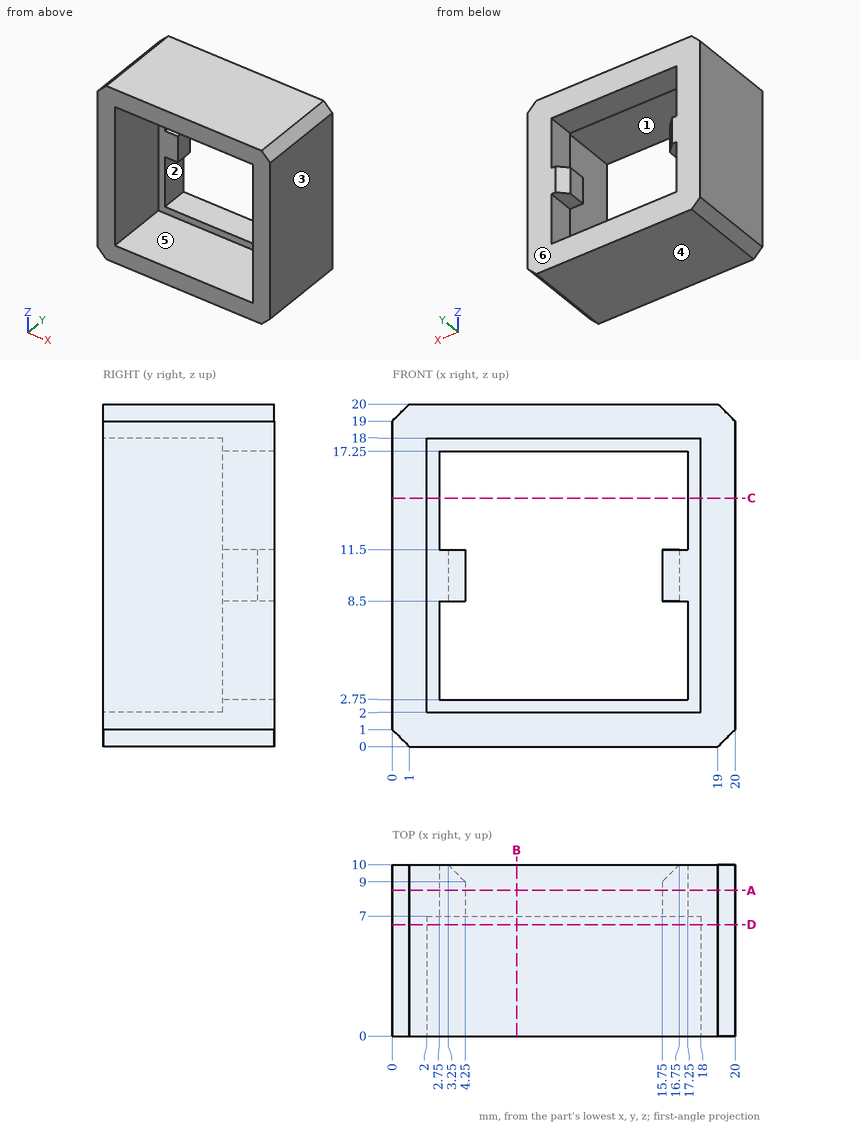
Part print with two shaded views. Sizes in mm from the minimum x, y, z corner. A direction names the side the tool comes from. Round coordinates to 2 decimals unless told otherwise and drop trailing zeros. Write each loop counter-clockwise with the first axis right and the second up, starting at its lowest first coordinate (ties: lowest second). Pieces come first, ordered by that corner, then holes. Notation, with made-up numbers: M 45,-9 L 52,-9 A18 cw 52,26 Z; hole C 66.25,77.5 d9. An arc over 180 degrees is marked long. Answer as CSV lines item,"result". Start each with the question number.
1) Mould opens along Z. For the marked faces 4, 5 and 6 say: +Z half, -Z half, draft (parallel to the pull), parting line (faces both ways), or undercut.
2) Drop a flat-ended pin along its axis: pin 1 (5 mm diameter, centred on x = 11.5, z = 12, fed in from -Y). Give the stop position or say it passes through.
3) Band-saw the part on C-C (z = 14.5). List the corners of the cut face in (x, y).
4) Band-saw the part on B-B (x = 7.25). List the corners of the cut face in (y, z).
5) Which spindle directions (+Z, -Z, +X, -X, +Y, -Y) get a long thin tool onto all of the face, cutting with end or side? Do the marked faces 1, 2 and 3. Say none if no direction does.
6) Band-saw the part on A-A (y = 8.5). List the corners of the cut face in (x, z).
7) Drill centre lines: L1, parallel to X at y = 8, z = 4.25; L2, parallel to X at y = 5.5, z = 8.75. Where is each one in solid material? Low to high.
8) Band-saw the part on D-D (y = 6.5). List the corners of the cut face in (x, z).
Worked out:
1,face 4,"-Z half"
1,face 5,"undercut"
1,face 6,"draft"
2,pin 1,"through"
3,outline,"M 0,0 L 2,0 L 2,7 L 2.75,7 L 2.75,10 L 0,10 Z; M 17.25,7 L 18,7 L 18,0 L 20,0 L 20,10 L 17.25,10 Z"
4,outline,"M 0,0 L 10,0 L 10,2.75 L 7,2.75 L 7,2 L 0,2 Z; M 0,18 L 7,18 L 7,17.25 L 10,17.25 L 10,20 L 0,20 Z"
5,face 1,"-Y"
5,face 2,"+Y, -Y"
5,face 3,"+Z, -Z, +X, +Y, -Y"
6,outline,"M 0,1 L 1,0 L 19,0 L 20,1 L 20,19 L 19,20 L 1,20 L 0,19 Z; hole M 2.75,2.75 L 17.25,2.75 L 17.25,8.5 L 15.75,8.5 L 15.75,11.5 L 17.25,11.5 L 17.25,17.25 L 2.75,17.25 L 2.75,11.5 L 4.25,11.5 L 4.25,8.5 L 2.75,8.5 Z"
7,L1,"0 to 2.75, 17.25 to 20"
7,L2,"0 to 2, 18 to 20"
8,outline,"M 0,1 L 1,0 L 19,0 L 20,1 L 20,19 L 19,20 L 1,20 L 0,19 Z; hole M 2,2 L 18,2 L 18,18 L 2,18 Z"
